Could you check a few things on this model? Use its own coordinates, in mm. A direction names the side the tool comes from. Round coordinates to 2 decimals unless told otherwise and drop trailing zeros. Loops run counter-clockwise (first coordinate to the right, second up) from the corner with the lowest first, then second, coordinate; pieces in that order, holes last.
from build123d import *

# Parameters (mm, degrees)
F0_W     = 204
F0_H     = 128
F0_W_2   = 166
F0_H_2   = 101
F0_W_3   = 12.5
F1_DEPTH = 5
F2_D     = 3.3
F4_D     = 3.3
F5_R     = 5


with BuildPart() as f1:
    # F0 (on Top) → F1 (new body)
    with BuildSketch(Plane.XY):
        with Locations((1, 0.5)):
            Rectangle(F0_W, F0_H)
        Rectangle(F0_W_2, F0_H_2, mode=Mode.SUBTRACT)
        with Locations((109.25, 0.5)):
            Rectangle(F0_W_3, F0_H)
    extrude(amount=F1_DEPTH)

    # F2 (through all)
    with Locations(Plane(origin=(0, 0, 0), x_dir=(1, 0, 0), z_dir=(0, 0, -1))):
        with Locations((-97, -60.5), (99, -60.5), (99, 59.5), (-97, 59.5)):
            Hole(F2_D / 2)

    # F4 (through all)
    with Locations(Plane.XY.offset(5)):
        with Locations((-87.9689130953, 51.0566890079), (87.853647545, 51.7008769748), (87.7295576794, -52.1221233483), (-87.9235801444, -51.3708378505)):
            Hole(F4_D / 2)

    # F5
    f5_edges = [f1.edges().sort_by_distance(p)[0] for p in [
        (-101, 64.5, 2.5),
        (115.5, 64.5, 2.5),
        (115.5, -63.5, 2.5),
        (-101, -63.5, 2.5),
    ]]
    fillet(f5_edges, radius=F5_R)


solid = f1.part
Item 1: If we section it at B-B, the plane x = -16: Please give me the cut outline in (y, z).
Results list:
outline: (-63.5, 0) - (-50.5, 0) - (-50.5, 5) - (-63.5, 5) - close; (50.5, 0) - (64.5, 0) - (64.5, 5) - (50.5, 5) - close
Item 2: Will this pin go through, and if not, where does the flat tip stop? pin 1 (3 mm diameter, centred on x = 99, y = -59.5, fed in from -Z).
Results list:
pin 1: passes through
Item 3: We'd pull the mould along Y, two halves only. Please class faces 3 (the flat face through (-83, -1, 2)), 4 (the cylindrical face through (-99.57, 63, 2.54)), 5 (the flat face through (6, -55, 0)): released by +Y, released by -Y, zero draft, split by the parting line, or undercut.
Results list:
face 3: undercut
face 4: released by +Y
face 5: zero draft
Item 4: For faces 1 (the flat face through (-1, -50.5, 2)), 2 (the flat face through (6, -55, 5)), which set-ups out of +Z, -Z, +X, -X, +Y, -Y let a thin tool reach every point of the face, with its end or its side?
Results list:
face 1: +Z, -Z
face 2: +Z, +X, -X, +Y, -Y
Item 5: If we section it at C-C, the plane z = 4.1: Count the separate pieces of the cut face and the enclosed holes in it, then the cut area to 3 significant figures.
Results list:
separate pieces: 1
enclosed holes: 9
area: 10,900 mm2
Item 6: If I drill on line 1 along Y through (x, z) = (99, 3.7); line 2 along X through (y, z) = (-15, 1.35); line 3 along Y through (x, z) = (-1.5, 3), over which ranges is the centre line in solid material (lowest first)?
Results list:
line 1: y = -63.5 to -61.15, -57.85 to 58.85, 62.15 to 64.5
line 2: x = -101 to -83, 83 to 115.5
line 3: y = -63.5 to -50.5, 50.5 to 64.5
Item 7: If we section it at A-A, the plane y = -19.5: Please give me the cut outline in (x, z), then the cut area to 4 significant figures.
Results list:
outline: (-101, 0) - (-83, 0) - (-83, 5) - (-101, 5) - close; (83, 0) - (115.5, 0) - (115.5, 5) - (83, 5) - close
area: 252.5 mm2
